from build123d import *

# Parameters (mm, degrees)
SKETCH1_R           = 1.5
BOSS_EXTRUDE1_DEPTH = 3
EXTRUDE_1_DEPTH     = 3
EXTRUDE_3_DEPTH     = 3
EXTRUDE_4_REACH     = 98.931


with BuildPart() as part:
    # Sketch1 → Boss-Extrude1 (new body)
    # profile 1 of 2: a face of its own
    with BuildSketch(Plane.XY):
        with BuildLine():
            Line((20.05, 5), (0, 5))
            ThreePointArc((0, 5), (-5, 0), (0, -5))
            Line((0, -5), (22, -5))
            Line((22, -5), (25.516973514, -3.553997369))
            ThreePointArc((25.516973514, -3.553997369), (26.624391141, 1.901317064), (22, 5))
            Line((22, 5), (20.05, 5))
        make_face()
        Circle(SKETCH1_R, mode=Mode.SUBTRACT)
        with Locations((22, 0)):
            Circle(SKETCH1_R, mode=Mode.SUBTRACT)
    # profile 2 of 2: a face of its own
    with BuildSketch(Plane.XY):
        with BuildLine():
            Line((46.409029503, 15.837507263), (20.05, 5))
            Line((20.05, 5), (22, 5))
            ThreePointArc((22, 5), (26.624391141, 1.901317064), (25.516973514, -3.553997369))
            Line((25.516973514, -3.553997369), (48.359029503, 5.837507263))
            Line((48.359029503, 5.837507263), (58.872830999, 10.16025367))
            Line((58.872830999, 10.16025367), (53.359871826, 12.67140304))
            Line((53.359871826, 12.67140304), (46.409029503, 15.837507263))
        make_face()
    extrude(amount=BOSS_EXTRUDE1_DEPTH)

    # 草图1 → 凸台-拉伸1 (add)
    with BuildSketch(Plane.XY.offset(3)):
        Polygon((46.409029503, 15.837507263), (58.872830999, 10.16025367), (111.008388469, 31.59577286), (98.544586973, 37.273026453), align=None)
    extrude(amount=-EXTRUDE_1_DEPTH)

    # 草图17 → 凸台-拉伸3 (add)
    with BuildSketch(Plane.XY.offset(3)):
        with BuildLine():
            Line((111.008388469, 31.59577286), (23.732077121, -4.287856999))
            Line((23.732077121, -4.287856999), (22.936363323, -2.318021512))
            ThreePointArc((22.936363323, -2.318021512), (24.318021512, 0.936363323), (21.063636677, 2.318021512))
            Line((21.063636677, 2.318021512), (19.990187108, 4.975407947))
            Line((19.990187108, 4.975407947), (98.544586973, 37.273026453))
            Line((98.544586973, 37.273026453), (111.008388469, 31.59577286))
        make_face()
    extrude(amount=EXTRUDE_3_DEPTH)

    # 凸台-拉伸4: up to this plane
    extrude_4_end = Plane(origin=(98.544586973, 37.273026453, -70.058401543), z_dir=(0.4145222599320868, 0.9100391727946636, 0))
    # 草图18 → 凸台-拉伸4 (add, up to the surface)
    with BuildSketch(Plane(origin=(18.913747522, 7.640196343, 0), x_dir=(0.3745453290899799, -0.9272086046067943, 0), z_dir=(0.9272086046067944, 0.37454532908997995, 0)), mode=Mode.PRIVATE) as extrude_4_sk1:
        with BuildLine():
            Line((13.499999459, -6), (13.499999459, -7))
            ThreePointArc((13.499999459, -7), (-4.500000541, -25), (13.499999459, -43))
            Line((13.499999459, -43), (13.499999459, -44))
            ThreePointArc((13.499999459, -44), (-4.669553865, -30.55583765), (2.873990149, -9.249192842))
            Line((2.873990149, -9.249192842), (2.873990149, -6))
            Line((2.873990149, -6), (13.499999459, -6))
        make_face()
    extrude_4_tool1 = split(extrude(extrude_4_sk1.sketch, amount=EXTRUDE_4_REACH, mode=Mode.PRIVATE), bisect_by=extrude_4_end, keep=Keep.BOTH, mode=Mode.PRIVATE)
    add(extrude_4_tool1.solids().sort_by_distance((20.149314, 4.581481, 7.624596))[0])


solid = part.part
Source: CAD feature listing. Evaluate the final solid. Frame: model axes, mm. A direction names the side the tool comes from. Coordinates: 2 decimals unless noted, no trailing zeros. Write each loop counter-clockwise with the first axis right and the second up, starting at its lowest first coordinate (ties: lowest second). Pieces come first, ordered by that corner, then holes. Notation, with made-up numbers: M -32,85.25 L -1,85.25 A29 ccw -1,111.25 Z; hole C 40,6.5 d4. An arc over 180 degrees is marked long. Use a Markdown table: item, result.
1) Reachability of faces 1 (the flat face through (59.04, 20.75, 7.65)), 2 (the cylindrical face through (20.5, 0.07, 1.48)), 3 (the flat face through (58.72, 20.9, 2.96)) from +Z, -Z, +X, -X, +Y, -Y: full face, straight path, thin tool, end or side. Return the list, or none.
Conclusion:
| item | result |
|---|---|
| face 1 | -X, +Y |
| face 2 | -Z |
| face 3 | -Z, -X, +Y |
2) Mould query, pull axis Y, two halves, no side actions, for faces 4 (the flat face through (53, 13, 0)), 5 (the flat face through (10, 5, 1)), 6 (the cylindrical face through (24.338, 0.885, 4.479)). Classes: pulls with the +Y half, pulls with the -Y half, needs draft (parallel to the pull), parting line crosses it, or undercut.
Conclusion:
| item | result |
|---|---|
| face 4 | needs draft |
| face 5 | pulls with the +Y half |
| face 6 | undercut |
3) Section B-B, the plane z = 28. Output: boundary loops of the cut face in (x, y).
Conclusion:
| item | result |
|---|---|
| outline | M 16.94,12.52 L 17.32,11.58 L 90.27,41.04 L 88.99,41.62 Z |
4) Ray query, L1, parallel to Y at x = 0, z = 1; L2, parallel to X at y = 0.5, z = 2; L3, parallel to Y at x = 22, z = 1.8. Return the intervals inside material, ascending.
Conclusion:
| item | result |
|---|---|
| L1 | y = -5 to -1.5, 1.5 to 5 |
| L2 | x = -4.97 to -1.41, 1.41 to 20.59, 23.41 to 35.38 |
| L3 | y = -5 to -1.5, 1.5 to 5.8 |
5) First-contact query: pin 1 Ø1.7 at (x, y) = (22, 0.5) entering from -Z; pin 2 Ø4 at (x, y) = (0, 0) entering from +Z; pin 3 Ø9.5 at (x, y) = (48.5, 16) entering from +Z. Flat tips, straight axial feed; report the tip coordinate or a pass-through.
Conclusion:
| item | result |
|---|---|
| pin 1 | stops at z = 6 |
| pin 2 | stops at z = 3 |
| pin 3 | stops at z = 43.21 |
6) Section A-A, the plane y = 0. Give the number of separate pieces and of enclosed holes in the cut face, then the cut area to 3 significant figures.
Conclusion:
| item | result |
|---|---|
| separate pieces | 4 |
| enclosed holes | 0 |
| area | 160 mm^2 |
